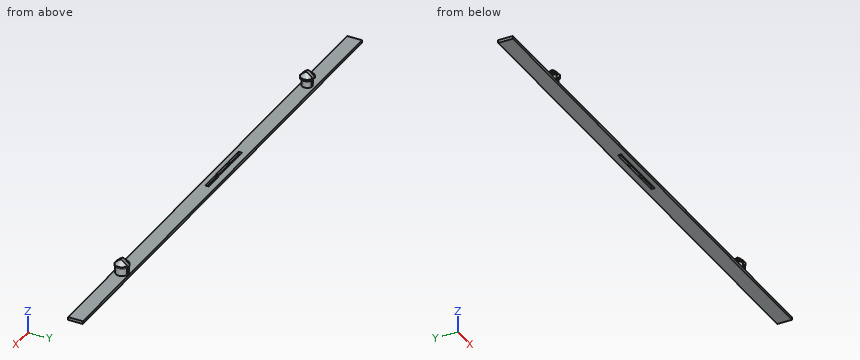
from build123d import *

# Parameters (mm, degrees)
SKICA2_W                 = 150
SKICA2_H                 = 4.2
SKICA2_W_2               = 18
SKICA2_H_2               = 1
P_IDAT_VYSUNUT_M2_DEPTH  = 0.8
SKICA3_R                 = 1.5
SKICA3_R_2               = 1.75
P_IDAT_VYSUNUT_M3_DEPTH  = 2.2
SKICA4_W                 = 0.6
SKICA4_H                 = 1
SKICA4_H_2               = 1.2
P_IDAT_VYSUNUT_M4_DEPTH  = 0.8
ZKOSEN_1_SIZE            = 0.4
ZKOSEN_1_SIZE2           = 0.145588094
ZKOSEN_1_PART_2_SIZE     = 0.4
ZKOSEN_1_PART_2_SIZE2    = 0.145588094
ZKOSEN_1_PART_3_SIZE     = 0.4
ZKOSEN_1_PART_3_SIZE2    = 0.145588094
ZKOSEN_1_PART_4_SIZE     = 0.4
ZKOSEN_1_PART_4_SIZE2    = 0.145588094
SKICA5_R                 = 1.9
P_IDAT_VYSUNUT_M5_DEPTH  = 2
ZKOSEN_2_SIZE            = 1.5
SKICA7_W                 = 1
SKICA7_H                 = 5
ODEBRAT_VYSUNUT_M1_DEPTH = 4


with BuildPart() as part:
    # Skica2 → Přidat vysunutím2 (new body)
    with BuildSketch(Plane.XY):
        Rectangle(SKICA2_W, SKICA2_H)
        with Locations((-5, -0.2)):
            Rectangle(SKICA2_W_2, SKICA2_H_2, mode=Mode.SUBTRACT)
    extrude(amount=P_IDAT_VYSUNUT_M2_DEPTH)

    # Skica3 → Přidat vysunutím3 (add)
    with BuildSketch(Plane.XY.offset(0.8)):
        with Locations((-50, -0.2)):
            Circle(SKICA3_R)
        with Locations((50, 0)):
            Circle(SKICA3_R_2)
    extrude(amount=P_IDAT_VYSUNUT_M3_DEPTH)

    # Skica4 → Přidat vysunutím4 (add)
    with BuildSketch(Plane(origin=(0, 0, 0), x_dir=(-1, 0, 0), z_dir=(0, 0, -1))):
        with Locations((1.9, -0.2)):
            Rectangle(SKICA4_W, SKICA4_H)
        with Locations((8.1, -0.1)):
            Rectangle(SKICA4_W, SKICA4_H_2)
    extrude(amount=-P_IDAT_VYSUNUT_M4_DEPTH)

    # Zkosení1
    zkosen_1_edges = [part.edges().sort_by_distance(p)[0] for p in [
        (-1.6, -0.2, 0),
    ]]
    zkosen_1_side = [part.faces().sort_by_distance(p)[0] for p in [
        (-1.6, -0.2, 0.4),
    ]]
    chamfer(zkosen_1_edges, length=ZKOSEN_1_SIZE, length2=ZKOSEN_1_SIZE2, reference=zkosen_1_side[0])

    # Zkosení1 part 2
    zkosen_1_part_2_edges = [part.edges().sort_by_distance(p)[0] for p in [
        (-2.2, -0.2, 0),
    ]]
    zkosen_1_part_2_side = [part.faces().sort_by_distance(p)[0] for p in [
        (-2.2, -0.2, 0.4),
    ]]
    chamfer(zkosen_1_part_2_edges, length=ZKOSEN_1_PART_2_SIZE, length2=ZKOSEN_1_PART_2_SIZE2, reference=zkosen_1_part_2_side[0])

    # Zkosení1 part 3
    zkosen_1_part_3_edges = [part.edges().sort_by_distance(p)[0] for p in [
        (-8.4, -0.2, 0),
    ]]
    zkosen_1_part_3_side = [part.faces().sort_by_distance(p)[0] for p in [
        (-8.4, -0.2, 0.4),
    ]]
    chamfer(zkosen_1_part_3_edges, length=ZKOSEN_1_PART_3_SIZE, length2=ZKOSEN_1_PART_3_SIZE2, reference=zkosen_1_part_3_side[0])

    # Zkosení1 part 4
    zkosen_1_part_4_edges = [part.edges().sort_by_distance(p)[0] for p in [
        (-7.8, -0.2, 0),
    ]]
    zkosen_1_part_4_side = [part.faces().sort_by_distance(p)[0] for p in [
        (-7.8, -0.2, 0.4),
    ]]
    chamfer(zkosen_1_part_4_edges, length=ZKOSEN_1_PART_4_SIZE, length2=ZKOSEN_1_PART_4_SIZE2, reference=zkosen_1_part_4_side[0])

    # Skica5 → Přidat vysunutím5 (add)
    with BuildSketch(Plane.XY.offset(3)):
        with Locations((-50, -0.2)):
            Circle(SKICA5_R)
        with Locations((50, 0)):
            Circle(SKICA5_R)
    extrude(amount=P_IDAT_VYSUNUT_M5_DEPTH)

    # Zkosení2
    zkosen_2_edges = [part.edges().sort_by_distance(p)[0] for p in [
        (-51.9, -0.2, 5),
        (48.1, 0, 5),
    ]]
    chamfer(zkosen_2_edges, length=ZKOSEN_2_SIZE)

    # Skica7 → Odebrat vysunutím1 (cut)
    with BuildSketch(Plane.XY.offset(5)):
        with Locations((-50, -0.2)):
            Rectangle(SKICA7_W, SKICA7_H)
        with Locations((50, 0)):
            Rectangle(SKICA7_W, SKICA7_H)
    extrude(amount=-ODEBRAT_VYSUNUT_M1_DEPTH, mode=Mode.SUBTRACT)


solid = part.part
Build history of the part. All positions in model axes, mm. Round coordinates to 2 decimals unless told otherwise and drop trailing zeros. Write each loop counter-clockwise with the first axis right and the second up, starting at its lowest first coordinate (ties: lowest second). Pieces come first, ordered by that corner, then holes. Notation, with made-up numbers: (-21, 4) - (-4, 4) arc R4 ccw to (-4, 11) - close; hole circle Ø1 at (61, -36). An arc over 180 degrees is marked (long way). Use CSV: the item, a comma, the result in double quotes.
(1) Band-saw the part on A-A (x = 64). Write the cut outline in (y, z).
Response:
outline,"(-2.1, 0) - (2.1, 0) - (2.1, 0.8) - (-2.1, 0.8) - close"
(2) Pin check, flat tips, straight feed: P1, Ø1, axis at x = -10, z = 1.5, coming from the +Y side; P2, Ø2, axis at y = 0, z = 3.5, coming from the +X side; P3, Ø2, axis at x = -6.5, y = 1, coming from the +Z side. Stop position of each tip, or through.
Response:
P1,"through"
P2,"x = 51.9"
P3,"z = 0.8"
(3) Wall check: line 1 (X direction, y = -0.3, z = 3.2); line 2 (X direction, y = 0.6, z = 3.7); line 3 (Z direction, x = -46, y = -1.65). Give the ranges that are in metal, low to high.
Response:
line 1,"-51.9 to -50.5, -49.5 to -48.1, 48.12 to 49.5, 50.5 to 51.88"
line 2,"-51.5 to -50.5, -49.5 to -48.5, 48.41 to 49.5, 50.5 to 51.59"
line 3,"0 to 0.8"
